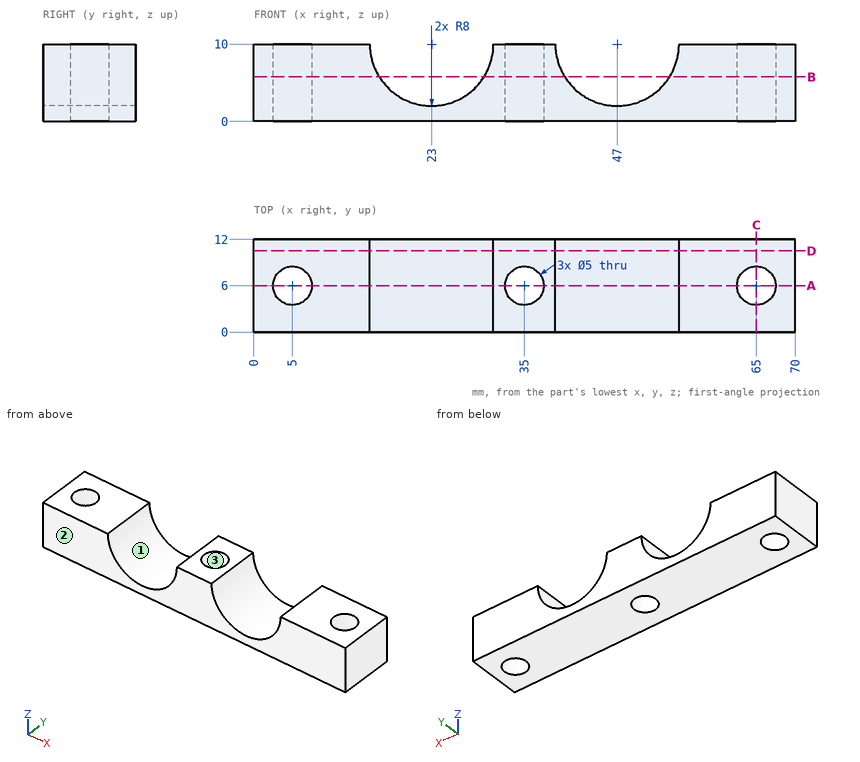
Design review of the part shown in the three views and the two pictorial views. Dimensions are in mm from the part's minimum x, y and z. Round coordinates to 2 decimals unless told otherwise and drop trailing zeros. Loops run counter-clockwise (first coordinate to the right, second up) from the corner with the lowest first, then second, coordinate; pieces in that order, holes last. Notation, with made-up numbers: (24.5, -24.5) -> (68.5, -24.5) arc R12 cw to (68.5, -19.5) -> close; hole circle Ø3 at (-33, -23.5). An arc over 180 degrees is marked (long way). Answer as a JSON object with one key per item and string values. Group by question number.
1) We need section D-D on y = 10.5. Write out the cut boundary in (x, z).
2) We need section C-C on x = 65. Write out the cut boundary in (y, z), then the cut area to 3 significant figures.
3) Mouldability with a two-part tool opening along Y and no side actions: class the marked faces 1, 2 and 3 as released by +Y, released by -Y, zero draft, split by the parting line, or undercut.
4) We need section B-B on z = 5.75. Write out the cut boundary in (x, y), then the cut area to 3 significant figures.
5) We need section A-A on y = 6. Write out the cut boundary in (x, z).
6) For pin 1 Ø5 at (x, z) = (28, 7.5) entering from -Y; pin 2 Ø3 at (x, y) = (18.5, 1.5) entering from +Z; pin 3 Ø2 at (x, z) = (18, 7) entering from +Y, all flat-tipped, find the tip position at first contact; note any pin that passes through.
7) For line 1 (Y direction, x = 5, z = 4.25); line 2 (X direction, y = 4, z = 6); line 3 (X direction, y = 5.75, z = 7.75), list the stretches that pass through material, from the lowest coordinate up. Write a range as [from, to].
Result set:
{
 "1": {"outline": "(0, 0) -> (70, 0) -> (70, 10) -> (55, 10) arc R8 cw to (39, 10) -> (31, 10) arc R8 cw to (15, 10) -> (0, 10) -> close"},
 "2": {"outline": "(0, 0) -> (3.5, 0) -> (3.5, 10) -> (0, 10) -> close; (8.5, 0) -> (12, 0) -> (12, 10) -> (8.5, 10) -> close", "area": "70.0 mm²"},
 "3": {"face 1": "zero draft", "face 2": "released by -Y", "face 3": "undercut"},
 "4": {"outline": "(0, 0) -> (16.22, 0) -> (16.22, 12) -> (0, 12) -> close; (29.78, 0) -> (40.22, 0) -> (40.22, 12) -> (29.78, 12) -> close; (53.78, 0) -> (70, 0) -> (70, 12) -> (53.78, 12) -> close; hole circle Ø5 at (5, 6); hole circle Ø5 at (35, 6); hole circle Ø5 at (65, 6)", "area": "456 mm²"},
 "5": {"outline": "(0, 0) -> (2.5, 0) -> (2.5, 10) -> (0, 10) -> close; (7.5, 0) -> (32.5, 0) -> (32.5, 10) -> (31, 10) arc R8 cw to (15, 10) -> (7.5, 10) -> close; (37.5, 0) -> (62.5, 0) -> (62.5, 10) -> (55, 10) arc R8 cw to (39, 10) -> (37.5, 10) -> close; (67.5, 0) -> (70, 0) -> (70, 10) -> (67.5, 10) -> close"},
 "6": {"pin 1": "y = 0", "pin 2": "z = 4.71", "pin 3": "through"},
 "7": {"line 1": "[0, 3.5], [8.5, 12]", "line 2": "[0, 3.5], [6.5, 16.07], [29.93, 33.5], [36.5, 40.07], [53.93, 63.5], [66.5, 70]", "line 3": "[0, 2.51], [7.49, 15.32], [30.68, 32.51], [37.49, 39.32], [54.68, 62.51], [67.49, 70]"}
}
